Check sheet for the modelled part. Datum: model origin and axes. Units: mm. A direction names the side the tool comes from. Give positions to 0.01 mm unless a question says otherwise; leave off trailing zeros. Order: outer loops, then holes, each group sorted by start corner. A loop starts at its lowest first (then second) coordinate and runs counter-clockwise, first axis right, second up.
Item 1: Release check for a two-part mould opening along Z. For faces 1 (the flat face through (0, 0, 0)), 2 (the cylindrical face through (27.54, 27.81, 5.88)), 3 (the flat face through (-30, 0, 5)), 4 (the flat face through (-25, 25, 5)) record: released by +Z, released by -Z, zero draft, split by the parting line, or undercut.
Item 2: Gauge pin test, flat ends, axial feed: P1, Ø8, axis at x = 17.5, y = -11, coming from the -Z side; P2, Ø5.5, axis at y = 25, z = 5, coming from the -X side; P3, Ø1.8, axis at y = -23.5, z = 4.5, coming from the +X side. Record the tip position at first contact, or that the pin passes through.
Item 3: Sectioned sample at C-C on y = 25. Record the boundary of the cut face in (x, z).
Item 4: Material ranges on line 1 along Z through (x, y) = (27.6, -25); line 2 along Z through (x, y) = (29, 25); line 3 along X through (y, z) = (23, 6.75), recorded low to high.
Item 5: Sectioned sample at B-B on z = 5. Record the boundary of the cut face in (x, y).
Item 6: Sectioned sample at A-A on y = -25. Record the boundary of the cut face in (x, z).
Item 7: Access from +Z, -Z, +X, -X, +Y, -Y to the whole of each face (thin tool, end or side, straight path). Record for faces 5 (the cylindrical face through (-27.54, -24.35, 2.07)), 6 (the flat face through (0, 0, 10)), 7 (the cylindrical face through (27.5, -27.4, 3.2)).
from build123d import *

# Parameters (mm, degrees)
F0_W     = 60
F0_H     = 60
F1_DEPTH = 10
F2_R     = 3
F2_R_2   = 2.943246
F4_DEPTH = 5
F3_R     = 3
F5_DEPTH = 5


with BuildPart() as f1:
    # F0 (on Top) → F1 (new body)
    with BuildSketch(Plane.XY):
        Rectangle(F0_W, F0_H)
    extrude(amount=F1_DEPTH)

    # F2 (on face) → F4 (cut)
    with BuildSketch(Plane.YZ.offset(30)):
        with Locations((-25, 5)):
            Circle(F2_R)
        with Locations((25, 5)):
            Circle(F2_R_2)
    extrude(amount=-F4_DEPTH, mode=Mode.SUBTRACT)

    # F3 (on face) → F5 (cut)
    with BuildSketch(Plane(origin=(-30, 0, 0), x_dir=(0, -1, 0), z_dir=(-1, 0, 0))):
        with Locations((-25, 5)):
            Circle(F3_R)
        with Locations((25, 5)):
            Circle(F3_R)
    extrude(amount=-F5_DEPTH, mode=Mode.SUBTRACT)


solid = f1.part
Report:
1. face 1: released by -Z
1. face 2: undercut
1. face 3: zero draft
1. face 4: undercut
2. P1: stops at z = 0
2. P2: stops at x = -25
2. P3: stops at x = 25
3. outline: (-30, 0) - (30, 0) - (30, 2.06) - (25, 2.06) - (25, 7.94) - (30, 7.94) - (30, 10) - (-30, 10) - (-30, 8) - (-25, 8) - (-25, 2) - (-30, 2) - close
4. line 1: z = 0 to 2, 8 to 10
4. line 2: z = 0 to 2.06, 7.94 to 10
4. line 3: x = -25 to 25
5. outline: (-30, -30) - (30, -30) - (30, -28) - (25, -28) - (25, -22) - (30, -22) - (30, 22.06) - (25, 22.06) - (25, 27.94) - (30, 27.94) - (30, 30) - (-30, 30) - (-30, 28) - (-25, 28) - (-25, 22) - (-30, 22) - (-30, -22) - (-25, -22) - (-25, -28) - (-30, -28) - close
6. outline: (-30, 0) - (30, 0) - (30, 2) - (25, 2) - (25, 8) - (30, 8) - (30, 10) - (-30, 10) - (-30, 8) - (-25, 8) - (-25, 2) - (-30, 2) - close
7. face 5: -X
7. face 6: +Z, +X, -X, +Y, -Y
7. face 7: +X
